Geometry: final body of the model. Coordinates: model frame, mm. Give positions to 0.01 mm unless a question says otherwise; leave off trailing zeros. Write each loop counter-clockwise with the first axis right and the second up, starting at its lowest first coordinate (ties: lowest second). Pieces come first, ordered by that corner, then holes.
Q1. Cut plane A-A on x = 0. Return the cut outline in (y, z).
Q2. Cut plane B-B on z = 1.5. Count the separate pieces of the cut face and the enclosed holes in it, plus the area to 3 significant figures.
Q3. Pin query (flat end, axial travel): pin 1 (1 mm diameter, centred on x = -1, z = 3.5, fed in from -Y). Return the tip coordinate at first contact, or that it passes through.
Q4. Cut plane C-C on x = 44. Return the cut outline in (y, z), plus the area to 3 significant figures.
Q5. Line query: L1, parallel to Y at x = 2, z = 1.25; L2, parallel to X at y = -15.5, z = 1.5; L3, parallel to Y at x = -29, z = 1.25. Output: solid intervals per line, ascending.
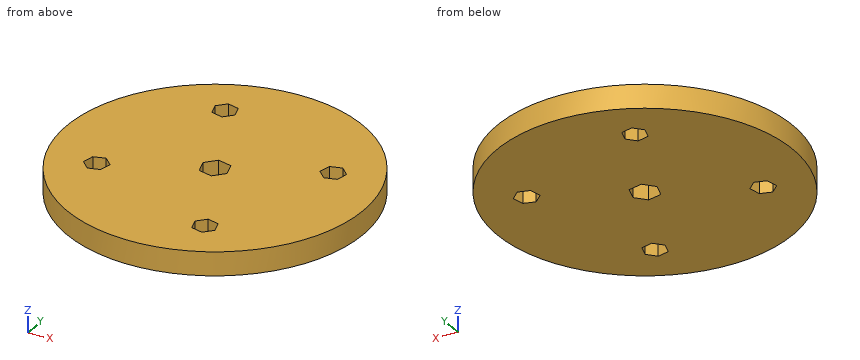
Autodesk Fusion 360 part; units mm, degrees
sketch "mainbase" plane through (0, 0, 0) normal (0, 0, 1) x (1, 0, 0)
  circle A0 centre (0, 0) radius 50
  circle A1 centre (0, 0) radius 46.5
  line L0 (-42.0315, -19.8897) -> (5.9278, -46.1206)
  line L1 (5.9278, -46.1206) -> (45.6951, -8.6144)
  line L2 (45.6951, -8.6144) -> (22.3133, 40.7966)
  line L3 (22.3133, 40.7966) -> (-31.9047, 33.8281)
  line L4 (-31.9047, 33.8281) -> (-42.0315, -19.8897)
  line L5 (-31.9047, 33.8281) -> (0, 0)
  line L6 (0, 0) -> (-42.0315, -19.8897)
  line L7 (5.9278, -46.1206) -> (0, 0)
  line L8 (45.6951, -8.6144) -> (0, 0)
  line L9 (22.3133, 40.7966) -> (0, 0)
  line L10 (-20.0354, 17.8663) -> (-16.8802, 20.3249)
  line L11 (-16.8802, 20.3249) -> (-17.4318, 24.2866)
  line L12 (-17.4318, 24.2866) -> (-21.1386, 25.7899)
  line L13 (-21.1386, 25.7899) -> (-24.2938, 23.3313)
  line L14 (-24.2938, 23.3313) -> (-23.7422, 19.3695)
  line L15 (-23.7422, 19.3695) -> (-20.0354, 17.8663)
  line L16 (19.2822, 26.9195) -> (19.1418, 30.9171)
  line L17 (19.1418, 30.9171) -> (15.6096, 32.7942)
  line L18 (15.6096, 32.7942) -> (12.2178, 30.6738)
  line L19 (12.2178, 30.6738) -> (12.3583, 26.6762)
  line L20 (12.3583, 26.6762) -> (15.8905, 24.7991)
  line L21 (15.8905, 24.7991) -> (19.2822, 26.9195)
  line L22 (30.8937, -9.0267) -> (34.6805, -10.315)
  line L23 (34.6805, -10.315) -> (37.6897, -7.6796)
  line L24 (37.6897, -7.6796) -> (36.912, -3.756)
  line L25 (36.912, -3.756) -> (33.1251, -2.4676)
  line L26 (33.1251, -2.4676) -> (30.116, -5.103)
  line L27 (30.116, -5.103) -> (30.8937, -9.0267)
  line L28 (8.3833, -33.8748) -> (6.093, -30.5954)
  line L29 (6.093, -30.5954) -> (2.1078, -30.9391)
  line L30 (2.1078, -30.9391) -> (0.4128, -34.5622)
  line L31 (0.4128, -34.5622) -> (2.7031, -37.8417)
  line L32 (2.7031, -37.8417) -> (6.6883, -37.498)
  line L33 (6.6883, -37.498) -> (8.3833, -33.8748)
  line L34 (-27.3524, -13.6107) -> (-30.2612, -10.865)
  line L35 (-30.2612, -10.865) -> (-34.0934, -12.0112)
  line L36 (-34.0934, -12.0112) -> (-35.0169, -15.9031)
  line L37 (-35.0169, -15.9031) -> (-32.1082, -18.6488)
  line L38 (-32.1082, -18.6488) -> (-28.2759, -17.5026)
  line L39 (-28.2759, -17.5026) -> (-27.3524, -13.6107)
  line L40 (1.4219, -4.5846) -> (4.6813, -1.0609)
  line L41 (4.6813, -1.0609) -> (3.2594, 3.5237)
  line L42 (3.2594, 3.5237) -> (-1.4219, 4.5846)
  line L43 (-1.4219, 4.5846) -> (-4.6813, 1.0609)
  line L44 (-4.6813, 1.0609) -> (-3.2594, -3.5237)
  line L45 (-3.2594, -3.5237) -> (1.4219, -4.5846)
  point P0 (-20.587, 21.8281)
  point P1 (15.75, 28.7966)
  point P2 (33.9028, -6.3913)
  point P3 (4.3981, -34.2185)
  point P4 (-31.1847, -14.7569)
  dimension "d1" = 100
  dimension "d2" = 93
  dimension "d3" = 46.5
  dimension "d4" = 4
  dimension "d5" = 12
  dimension "d6" = 4
  dimension "d7" = 12
  dimension "d8" = 4
  dimension "d9" = 12
  dimension "d10" = 4
  dimension "d11" = 12
  dimension "d12" = 4
  dimension "d13" = 12
  dimension "d14" = 4.8
extrude "Extrude1" add sketch "mainbase" along normal blind 8 contours A0 | A1 L2 | A1 L3 | L3 L5 L9 L10 L11 L12 L13 L17 L18 L19 L20 L42 L43 | L2 L8 L9 L16 L17 L20 L21 L24 L25 L26 L27 L41 L42 | A1 L1 | L1 L7 L8 L22 L23 L24 L27 L28 L29 L32 L33 L40 L41 L45 | A1 L4 | L4 L5 L6 L10 L13 L14 L15 L34 L35 L36 L37 L43 L44 | L9 L16 L17 L20 L21 | L9 L17 L18 L19 L20 | A1 L0 | L0 L6 L7 L29 L30 L31 L32 L34 L37 L38 L39 L44 L45 | L8 L22 L23 L24 L27 | L8 L24 L25 L26 L27 | L5 L10 L11 L12 L13 | L5 L10 L13 L14 L15 | L7 L29 L30 L31 L32 | L7 L28 L29 L32 L33 | L6 L34 L35 L36 L37 | L6 L34 L37 L38 L39
extrude "Extrude2" cut sketch "mainbase" along normal blind 25 contours L6 L34 L35 L36 L37 | L6 L34 L37 L38 L39
pattern_circular "C-Pattern1" count 4 over 360 about axis through (0, 0, 1.75) along (0, 0, 1) of "Extrude2"
equation "d3 = ( 93 / 2 ) * 1 mm"
Data:
1. outline: (-50, 0) - (-4.26, 0) - (-4.26, 8) - (-50, 8) - close; (4.26, 0) - (50, 0) - (50, 8) - (4.26, 8) - close
2. separate pieces: 1
2. enclosed holes: 5
2. area: 7,630 mm2
3. pin 1: stops at y = -50
4. outline: (-23.75, 0) - (23.75, 0) - (23.75, 8) - (-23.75, 8) - close
4. area: 380 mm2
5. L1: y = -49.96 to -3.96, 3.81 to 49.96
5. L2: x = -47.54 to -34.92, -27.8 to 47.54
5. L3: y = -40.73 to -17.72, -12.06 to 40.73
